Input: part model. Units: mm. Frame: model coordinates. A direction names the side the tool comes from. Round coordinates to 2 decimals unless told otherwise and drop trailing zeros. Order: outer loops, then holes, each group sorted by start corner. A loop starts at its lowest first (then second) coordinate and runs counter-clockwise, first axis right, second up. Notation, with made-up numbers: (-26.5, 29) - (25.5, 29) arc R30 ccw to (25.5, 57) - close; hole circle Ø9 at (-9, 30.25). An arc over 180 degrees is marked (long way). One line per item, written item: value. Start each with the question number.
from build123d import *

# Parameters (mm, degrees)
SKETCH1_R           = 28
SKETCH1_R_2         = 16
BOSS_EXTRUDE1_DEPTH = 56
BOSS_EXTRUDE2_START = -24
BOSS_EXTRUDE2_DEPTH = 24
SKETCH5_R           = 16
CUT_EXTRUDE2_DEPTH  = 40


with BuildPart() as part:
    # Sketch1 → Boss-Extrude1 (new body)
    with BuildSketch(Plane(origin=(0, 0, 0), x_dir=(1, 0, 0), z_dir=(0, 1, 0))):
        with Locations(Location((0, 0, 0), (0, 0, 270))):
            Circle(SKETCH1_R)
        with Locations(Location((0, 0, 0), (0, 0, 270))):
            Circle(SKETCH1_R_2, mode=Mode.SUBTRACT)
    extrude(amount=BOSS_EXTRUDE1_DEPTH)

    # Sketch3 → Boss-Extrude2 (add)
    with BuildSketch(Plane(origin=(0, 56, 0), x_dir=(1, 0, 0), z_dir=(0, 1, 0)).offset(BOSS_EXTRUDE2_START)):
        with BuildLine():
            Line((-24, 90), (24, 90))
            Line((24, 90), (24, 14.422205102))
            ThreePointArc((24, 14.422205102), (0, 28), (-24, 14.422205102))
            Line((-24, 14.422205102), (-24, 90))
        make_face()
    extrude(amount=BOSS_EXTRUDE2_DEPTH)

    # Sketch5 → Cut-Extrude2 (cut)
    with BuildSketch(Plane(origin=(0, 0, -90), x_dir=(-1, 0, 0), z_dir=(0, 0, -1))):
        with Locations((0, 32)):
            Circle(SKETCH5_R)
    extrude(amount=-CUT_EXTRUDE2_DEPTH, mode=Mode.SUBTRACT)


solid = part.part
1. Set-up query: faces 4 (the face through (-15.62, 27.61, -3.47)), 5 (the face through (-24, 44, -52)), 6 (the face through (0, 48, -70)). Return all of +Z, -Z, +X, -X, +Y, -Y with unobstructed straight access to the full face (end or side cutting, diameter ignored); none if empty.
2. Section C-C (x = 0). Return the cut outline in (y, z), then the cut area to 3 significant figures.
3. Section A-A (z = 0). Return the cut outline in (x, y).
4. Section B-B (y = 42). Return the cut outline in (x, z).
5. Pin query (flat end, axial travel): pin 1 (3 mm diameter, centred on x = -11, y = 18, fed in from -Z); pin 2 (19 mm diameter, centred on y = 41, z = -37, fed in from +X); pin 3 (1.5 mm diameter, centred on x = -5.5, y = 18.5, fed in from +Z). Return the tip coordinate at first contact, or that it passes through.
6. Line query: line 1 (X direction, y = 35, z = 0); line 2 (X direction, y = 32.5, z = -83); line 3 (Y direction, x = 12.5, z = -40). Output: solid intervals per line, ascending. Write a range as from..to.
7. Pull-direction query (X, two-part tool) for faces 1 (the face through (-10.724, 27.608, 25.865)), 2 (the face through (0, 38, -50)), 3 (the face through (24, 44, -53)); classes: released by +X, released by -X, zero draft, split by the parting line, or undercut.
8. Section D-D (z = -73). Return the cut outline in (x, y).
Solved:
1. face 4: +Y, -Y
1. face 5: -Z, -X, +Y, -Y
1. face 6: -Z, -Y
2. outline: (0, -28) - (32, -28) - (32, -50) - (48, -50) - (48, -90) - (56, -90) - (56, -16) - (0, -16) - close; (0, 16) - (56, 16) - (56, 28) - (0, 28) - close
2. area: 2,190 mm²
3. outline: (-28, 0) - (-16, 0) - (-16, 56) - (-28, 56) - close; (16, 0) - (28, 0) - (28, 56) - (16, 56) - close
4. outline: (-24, -90) - (-12.49, -90) - (-12.49, -50) - (12.49, -50) - (12.49, -90) - (24, -90) - (24, -14.42) arc R28 ccw (long way) to (-24, -14.42) - close; hole circle Ø32 at (0, 0)
5. pin 1: stops at z = -26.34
5. pin 2: stops at x = 24
5. pin 3: stops at z = 27.59
6. line 1: x = -28..-16, 16..28
6. line 2: x = -24..-15.99, 15.99..24
6. line 3: y = 32..56
7. face 1: split by the parting line
7. face 2: undercut
7. face 3: released by +X
8. outline: (-24, 32) - (-16, 32) arc R16 cw to (16, 32) - (24, 32) - (24, 56) - (-24, 56) - close
